Part model, mm, in its own coordinate system. A direction names the side the tool comes from. Give positions to 0.01 mm unless a question says otherwise; leave off trailing zeros. Write each loop counter-clockwise with the first axis right and the second up, starting at its lowest first coordinate (ties: lowest second). Pieces come first, ordered by that corner, then holes. Notation, with made-up numbers: (-27.5, -5) - (-2.5, -5) arc R33 ccw to (-2.5, 26) - close; hole circle Ø10 at (75.5, -19). An arc over 180 degrees is marked (long way). Answer in a Markdown table with one row per item. Add a question column.
1. Band-saw the part on C-C on x = 15.5. Write the cut outline in (y, z), plus the area to 3 significant figures.
2. Band-saw the part on D-D on z = 16. Write the cut outline in (x, y), plus the area to 3 significant figures.
3. Band-saw the part on B-B on z = 3.5. Write the cut outline in (x, y), plus the area to 3 significant figures.
4. Band-saw the part on A-A on x = 0. Write the cut outline in (y, z).
5. Which spindle directions (+Z, -Z, +X, -X, +Y, -Y) get a long thin tool onto all of the face, cutting with end or side? Do faces 1 (the cylindrical face through (35, 18, 5)), 2 (the flat face through (-9, 31, 6)), 3 (the flat face through (31, 25, 6)). Say none if no direction does.
6. Probe line 1 along Y through (x, z) = (15.5, 1.65); line 2 along Z through (x, y) = (-35, 1.6); line 3 along X through (y, z) = (15, 10.75). List the from-to ranges inside material, lowest first.
7. Drop flat-ended pins along their axis: pin 1 Ø7.5 at (x, z) = (38.5, 13.5) entering from +Y; pin 2 Ø8 at (y, z) = (27.5, 11.5) entering from +X; pin 3 Ø2 at (y, z) = (8.5, 10) entering from -X; pin 4 Ø4.5 at (x, z) = (-35, 10) entering from -Y. Give the stop position or say it passes through.
8. Pull direction Y, two halves, no side cores. Call faces 4 (the flat face through (-33, 3, 20)), 5 (the cylindrical face through (16.39, 37.89, 2.96)), 6 (the flat face through (-27, 7, 14)): released by +Y, released by -Y, zero draft, split by the parting line, or undercut.
```python
from build123d import *

# Parameters (mm, degrees)
BOX001_W                             = 10
BOX001_H                             = 20
BOX001_DEPTH                         = 20
EXTRUDE002_DEPTH                     = 10
EXTRUDE002_ONTO_SKETCH003_ROLL_ANGLE = 90
BOX_W                                = 28.5
BOX_H                                = 5
BOX_DEPTH                            = 20
CLONE_PLACEMENT_ANGLE                = 180
CYLINDER_R                           = 5
CYLINDER_DEPTH                       = 35
CYLINDER_ROLL_ANGLE                  = -90
SKETCH_R                             = 1.65
SKETCH_R_2                           = 13
EXTRUDE_DEPTH                        = 6
EXTRUDE001_DEPTH                     = 4.5
CHAMFER_SIZE                         = 3
FILLET_1_R                           = 3
FILLET_2_R                           = 2
FILLET_3_R                           = 1


with BuildPart() as cubo:
    # Box001 → Box001 (new body)
    with BuildSketch(Plane(origin=(45, 0, 0), x_dir=(1, 0, 0), z_dir=(0, 0, 1))):
        with Locations((5, 10)):
            Rectangle(BOX001_W, BOX001_H)
    extrude(amount=BOX001_DEPTH)


with BuildPart() as clone_of_cubo:
    # Clone004 base: copy of Cubo
    add(cubo.part)


with BuildPart() as clone_of_cubo_1:
    # Clone004 placement: moved
    add(clone_of_cubo.part.moved(Location((-100, 0, 0))))


with BuildPart() as obj1:
    # Fusion002 base: copy of Cubo
    add(cubo.part)

    # Fusion002: union Clone of Cubo
    add(clone_of_cubo_1.part)


with BuildPart() as obj2:
    # Sketch003 as drawn → Extrude002 (new)
    with BuildSketch(Plane.XY):
        with BuildLine():
            ThreePointArc((-1.895057, 1.895035), (0, -2.68), (1.895057, 1.895035))
            Line((1.110092, 2.68), (1.895057, 1.895035))
            Line((-1.110092, 2.68), (1.110092, 2.68))
            Line((-1.895057, 1.895035), (-1.110092, 2.68))
        make_face()
    extrude(amount=-EXTRUDE002_DEPTH)


with BuildPart() as obj2_1:
    # Extrude002 onto Sketch003 roll: moved
    add(obj2.part.rotate(Axis((0, 0, 0), (1, 0, 0)), EXTRUDE002_ONTO_SKETCH003_ROLL_ANGLE))


with BuildPart() as obj2_2:
    # Extrude002 onto Sketch003 placement: moved
    add(obj2_1.part.moved(Location((0, 0, 10))))


with BuildPart() as obj2_3:
    # Extrude002 placement: moved
    add(obj2_2.part.moved(Location((35, -1, 0))))


with BuildPart() as clone002:
    # Clone002 base: copy of obj2
    add(obj2_3.part)


with BuildPart() as clone002_1:
    # Clone002 placement: moved
    add(clone002.part.moved(Location((-70, 0, 0))))


with BuildPart() as soporte_vertical:
    # Box → Box (new body)
    with BuildSketch(Plane(origin=(-50, 0, 0), x_dir=(1, 0, 0), z_dir=(0, 0, 1))):
        with Locations((14.25, 2.5)):
            Rectangle(BOX_W, BOX_H)
    extrude(amount=BOX_DEPTH)


with BuildPart() as cut:
    # Cut base: copy of soporte_vertical
    add(soporte_vertical.part)

    # Cut: cut Clone002
    add(clone002_1.part, mode=Mode.SUBTRACT)


with BuildPart() as cut001:
    # Clone base: copy of soporte_vertical
    add(soporte_vertical.part)


with BuildPart() as cut001_1:
    # Clone placement: moved
    add(cut001.part.moved(Location((0, 5, 0))).rotate(Axis((0, 5, 0), (0, 0, 1)), CLONE_PLACEMENT_ANGLE))

    # Cut001: cut obj2
    add(obj2_3.part, mode=Mode.SUBTRACT)


with BuildPart() as hueco_cabeza_tornillo:
    # Cylinder → Cylinder (new body)
    with BuildSketch(Plane.XY):
        Circle(CYLINDER_R)
    extrude(amount=CYLINDER_DEPTH)


with BuildPart() as hueco_cabeza_tornillo_1:
    # Cylinder roll: moved
    add(hueco_cabeza_tornillo.part.rotate(Axis((0, 0, 0), (1, 0, 0)), CYLINDER_ROLL_ANGLE))


with BuildPart() as hueco_cabeza_tornillo_2:
    # Cylinder placement: moved
    add(hueco_cabeza_tornillo_1.part.moved(Location((35, 5, 10))))


with BuildPart() as huecos_cabeza_tornillo:
    # Clone003 base: copy of hueco_cabeza_tornillo
    add(hueco_cabeza_tornillo_2.part)


with BuildPart() as huecos_cabeza_tornillo_1:
    # Clone003 placement: moved
    add(huecos_cabeza_tornillo.part.moved(Location((-70, 0, 0))))

    # Fusion: union hueco_cabeza_tornillo
    add(hueco_cabeza_tornillo_2.part)


with BuildPart() as base_hueco_motor_con_cabeza_tornillo:
    # Sketch → Extrude (new body)
    with BuildSketch(Plane.XY):
        Polygon((-30, 42), (30, 42), (50, 0), (-50, 0), align=None)
        with Locations((-15.5, 36.5)):
            Circle(SKETCH_R, mode=Mode.SUBTRACT)
        with Locations((15.5, 36.5)):
            Circle(SKETCH_R, mode=Mode.SUBTRACT)
        with Locations((-15.5, 5.5)):
            Circle(SKETCH_R, mode=Mode.SUBTRACT)
        with Locations((15.5, 5.5)):
            Circle(SKETCH_R, mode=Mode.SUBTRACT)
        with Locations((0, 21)):
            Circle(SKETCH_R_2, mode=Mode.SUBTRACT)
    extrude(amount=EXTRUDE_DEPTH)

    # Cut002: cut huecos_cabeza_tornillo
    add(huecos_cabeza_tornillo_1.part, mode=Mode.SUBTRACT)


with BuildPart() as obj3:
    # Sketch002 → Extrude001 (new body)
    with BuildSketch(Plane.YZ):
        Polygon((5, 20), (42, 6), (5, 6), align=None)
    extrude(amount=EXTRUDE001_DEPTH)


with BuildPart() as obj3_1:
    # Extrude001 placement: moved
    add(obj3.part.moved(Location((21.5, 0, 0))))


with BuildPart() as clone001:
    # Clone001 base: copy of obj3
    add(obj3_1.part)


with BuildPart() as clone001_1:
    # Clone001 placement: moved
    add(clone001.part.moved(Location((-47.5, 0, 0))))


with BuildPart() as nema17_holder_v03:
    # Fusion001 base: copy of obj3
    add(obj3_1.part)

    # Fusion001: union Cut, Cut001, base_hueco_motor_con_cabeza_tornillo, Clone001
    add(cut.part)
    add(cut001_1.part)
    add(base_hueco_motor_con_cabeza_tornillo.part)
    add(clone001_1.part)

    # Chamfer
    chamfer_edges = [nema17_holder_v03.edges().sort_by_distance(p)[0] for p in [
        (26, 5, 13),
        (26, 23.5, 6),
        (42.809524, 5, 6),
        (29, 5, 6),
        (-26, 23.5, 6),
        (-29, 5, 6),
        (-42.809524, 5, 6),
        (-26, 5, 13),
    ]]
    chamfer(chamfer_edges, length=CHAMFER_SIZE)

    # Cut003: cut obj1
    add(obj1.part, mode=Mode.SUBTRACT)

    # Fillet 1
    fillet_1_edges = [nema17_holder_v03.edges().sort_by_distance(p)[0] for p in [
        (45, 0, 10),
        (-45, 0, 10),
    ]]
    fillet(fillet_1_edges, radius=FILLET_1_R)

    # Fillet 2
    fillet_2_edges = [nema17_holder_v03.edges().sort_by_distance(p)[0] for p in [
        (45, 10.5, 3),
        (-45, 10.5, 3),
    ]]
    fillet(fillet_2_edges, radius=FILLET_2_R)

    # Fillet 3
    fillet_3_edges = [nema17_holder_v03.edges().sort_by_distance(p)[0] for p in [
        (30, 42, 3),
        (-30, 42, 3),
    ]]
    fillet(fillet_3_edges, radius=FILLET_3_R)


solid = nema17_holder_v03.part
```
Values:
| question | item | result |
|---|---|---|
| 1 | outline | (0, 0) - (3.85, 0) - (3.85, 6) - (0, 6) - close; (7.15, 0) - (34.85, 0) - (34.85, 6) - (7.15, 6) - close; (38.15, 0) - (42, 0) - (42, 6) - (38.15, 6) - close |
| 1 | area | 212 mm² |
| 2 | outline | (-45, 3) arc R3 ccw to (-42, 0) - (-21.5, 0) - (-21.5, 15.57) - (-26, 15.57) - (-26, 8) - (-29, 5) - (-45, 5) - close; (21.5, 0) - (42, 0) arc R3 ccw to (45, 3) - (45, 5) - (29, 5) - (26, 8) - (26, 15.57) - (21.5, 15.57) - close |
| 2 | area | 335 mm² |
| 3 | outline | (-45, 3) arc R3 ccw to (-42, 0) - (42, 0) arc R3 ccw to (45, 3) - (45, 10.05) arc R2 ccw to (44.81, 10.91) - (30.27, 41.43) arc R1 ccw to (29.37, 42) - (-29.37, 42) arc R1 ccw to (-30.27, 41.43) - (-44.81, 10.91) arc R2 ccw to (-45, 10.05) - close; hole circle Ø3.3 at (-15.5, 5.5); hole circle Ø3.3 at (-15.5, 36.5); hole circle Ø26 at (0, 21); hole circle Ø3.3 at (15.5, 5.5); hole circle Ø3.3 at (15.5, 36.5) |
| 3 | area | 2,740 mm² |
| 4 | outline | (0, 0) - (8, 0) - (8, 6) - (0, 6) - close; (34, 0) - (42, 0) - (42, 6) - (34, 6) - close |
| 5 | face 1 | +Z, +Y |
| 5 | face 2 | +Z, +Y, -Y |
| 5 | face 3 | +Z, +X, +Y |
| 6 | line 1 | y = 0 to 3.85, 7.15 to 34.85, 38.15 to 42 |
| 6 | line 2 | z = 0 to 7.32, 12.68 to 20 |
| 6 | line 3 | x = -26 to -21.5, 21.5 to 26 |
| 7 | pin 1 | stops at y = 5 |
| 7 | pin 2 | stops at x = 27.5 |
| 7 | pin 3 | stops at x = -26.5 |
| 7 | pin 4 | passes through |
| 8 | face 4 | zero draft |
| 8 | face 5 | undercut |
| 8 | face 6 | released by +Y |
